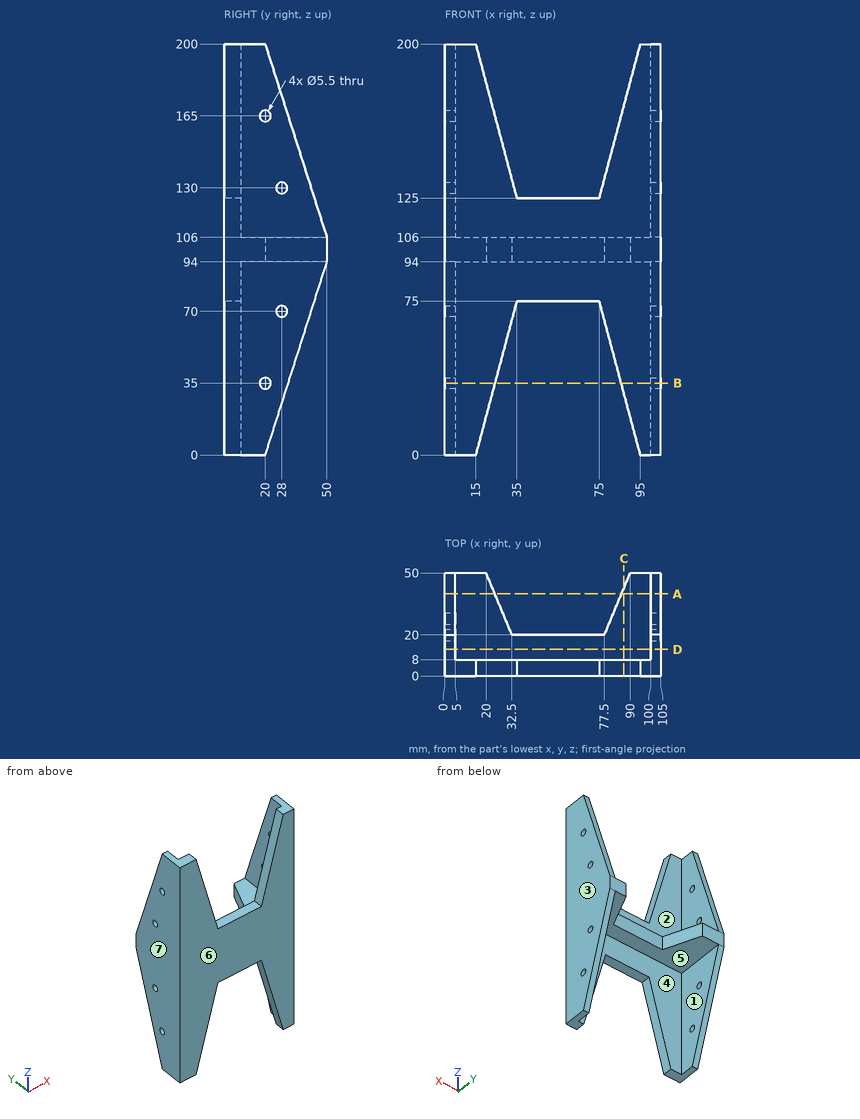
Could you check a few things on this drawing? It's one solid part, dimensions in mm from its lowest x, y, z. A direction names the side the tool comes from. Give positions to 0.01 mm unless a question says otherwise; leave off trailing zeros. Write each loop counter-clockwise with the first axis right and the second up, starting at its lowest first coordinate (ties: lowest second). Pieces come first, ordered by that corner, then holes. Notation, with made-up numbers: (-15, -26) - (40, -26) arc R10 ccw to (40, -11) - close; hole circle Ø4 at (64, -3.5). An arc over 180 degrees is marked (long way). Use CSV: the item, a comma, the result in double quotes. Start each with the question number.
Item 1: If we mould it in two halves opening along X, with no side actions, what happens to the marked faces 4, 5, 6 and 7? For each: pulls with the +X half, pulls with the -X half, needs draft (parallel to the pull), parting line crosses it, or undercut.
Item 2: I want a section at A-A, the plane y = 40. Please give me the cut outline in (x, z), then the cut area to 3 significant figures.
Item 3: I want a section at D-D, the plane y = 13. Please give me the cut outline in (x, z).
Item 4: If I drill on line 1 along X through (y, z) = (22, 146); line 2 along Z through (x, y) = (94, 30); line 3 along Y through (x, z) = (13, 42), over which ranges is the centre line in solid material (lowest first)?
Item 5: I'm going to push flat-ended pins straight in: pin 1 (1.5 mm diameter, centred on x = 93.5, y = 22, fed in from +Z); pin 2 (4 mm diameter, centred on x = 90, y = 41, fed in from -Z). Where does each tip first touch, or does it pass through?
Item 6: For the marked faces 1, 2 and 3, which set-ups out of +Z, -Z, +X, -X, +Y, -Y let a thin tool reach every point of the face, with its end or its side?
Item 7: I want a section at B-B, the plane z = 35. Please give me the cut outline in (x, y), then the cut area to 3 significant figures.
Item 8: I want a section at C-C, the plane x = 87. Please give me the cut outline in (y, z), then the cut area to 3 significant figures.
Findings:
1,face 4,"undercut"
1,face 5,"undercut"
1,face 6,"needs draft"
1,face 7,"pulls with the -X half"
2,outline,"(0, 62.67) - (5, 62.67) - (5, 94) - (24.17, 94) - (24.17, 106) - (5, 106) - (5, 137.33) - (0, 137.33) - close; (85.83, 94) - (100, 94) - (100, 62.67) - (105, 62.67) - (105, 137.33) - (100, 137.33) - (100, 106) - (85.83, 106) - close"
2,area,"1,150 mm2"
3,outline,"(0, 0) - (5, 0) - (5, 94) - (100, 94) - (100, 0) - (105, 0) - (105, 200) - (100, 200) - (100, 106) - (5, 106) - (5, 200) - (0, 200) - close"
4,line 1,"x = 0 to 5, 100 to 105"
4,line 2,"z = 94 to 106"
4,line 3,"y = 0 to 8"
5,pin 1,"stops at z = 106"
5,pin 2,"stops at z = 94"
6,face 1,"-Z, +Y"
6,face 2,"+Z, +Y"
6,face 3,"+Z, -Z, +X, +Y, -Y"
7,outline,"(0, 0) - (24.33, 0) - (24.33, 8) - (5, 8) - (5, 17.25) - (0, 17.25) - close; (0, 22.75) - (5, 22.75) - (5, 31.17) - (0, 31.17) - close; (85.67, 0) - (105, 0) - (105, 17.25) - (100, 17.25) - (100, 8) - (85.67, 8) - close; (100, 22.75) - (105, 22.75) - (105, 31.17) - (100, 31.17) - close"
7,area,"526 mm2"
8,outline,"(0, 30) - (8, 30) - (8, 94) - (42.8, 94) - (42.8, 106) - (8, 106) - (8, 170) - (0, 170) - close"
8,area,"1,540 mm2"
